from build123d import *

# Parameters (mm, degrees)
SKETCH1_W           = 50
SKETCH1_H           = 55
BOSS_EXTRUDE1_DEPTH = 5
SKETCH2_W           = 50
SKETCH2_H           = 70
BOSS_EXTRUDE2_DEPTH = 5
SKETCH3_W           = 50
SKETCH3_H           = 8
BOSS_EXTRUDE3_DEPTH = 50
FILLET1_R           = 2


with BuildPart() as part:
    # Sketch1 → Boss-Extrude1 (new body)
    with BuildSketch(Plane.XY):
        with Locations((-25, 27.5)):
            Rectangle(SKETCH1_W, SKETCH1_H)
    extrude(amount=BOSS_EXTRUDE1_DEPTH)

    # Sketch2 → Boss-Extrude2 (add)
    with BuildSketch(Plane(origin=(0, 0, 0), x_dir=(1, 0, 0), z_dir=(0, 1, 0))):
        with Locations((-25, -2.5)):
            Rectangle(SKETCH2_W, SKETCH2_H)
    extrude(amount=-BOSS_EXTRUDE2_DEPTH)

    # Sketch3 → Boss-Extrude3 (add)
    with BuildSketch(Plane(origin=(0, -5, 0), x_dir=(-1, 0, 0), z_dir=(0, -1, 0))):
        with Locations((25, -33.5)):
            Rectangle(SKETCH3_W, SKETCH3_H)
        with Locations((25, 28.5)):
            Rectangle(SKETCH3_W, SKETCH3_H)
    extrude(amount=BOSS_EXTRUDE3_DEPTH)

    # Fillet1
    fillet1_edges = [part.edges().sort_by_distance(p)[0] for p in [
        (-50, 0, 21.25),
        (-25, 0, 37.5),
        (0, 0, 21.25),
        (-50, -27.5, 37.5),
        (-50, -27.5, -32.5),
        (0, -27.5, -32.5),
        (0, -27.5, 37.5),
        (-50, 0, -16.25),
        (0, 0, -16.25),
        (-25, 0, -32.5),
        (0, -5, 2.5),
        (-50, -30, 29.5),
        (0, -55, 33.5),
        (0, -30, 29.5),
        (-25, -55, 37.5),
        (-25, -55, 29.5),
        (-50, -55, 33.5),
        (-50, -5, 2.5),
        (-25, -55, -24.5),
        (0, -30, -24.5),
        (-50, -55, -28.5),
        (-50, -30, -24.5),
        (-25, -55, -32.5),
        (0, -55, -28.5),
    ]]
    fillet(fillet1_edges, radius=FILLET1_R)


solid = part.part
Work out the finished part from the listing and answer in its coordinate system (mm). A direction names the side the tool comes from. Coordinates: 2 decimals unless noted, no trailing zeros. Write each loop counter-clockwise with the first axis right and the second up, starting at its lowest first coordinate (ties: lowest second). Pieces come first, ordered by that corner, then holes.
1. The part is cut by section A-A, the plane y = -20. Write down the section's boundary in (x, z), and give its area (3 significant figures).
Results list:
outline: (-50, -30.5) arc R2 ccw to (-48, -32.5) - (-2, -32.5) arc R2 ccw to (0, -30.5) - (0, -26.5) arc R2 ccw to (-2, -24.5) - (-48, -24.5) arc R2 ccw to (-50, -26.5) - close; (-50, 31.5) arc R2 ccw to (-48, 29.5) - (-2, 29.5) arc R2 ccw to (0, 31.5) - (0, 35.5) arc R2 ccw to (-2, 37.5) - (-48, 37.5) arc R2 ccw to (-50, 35.5) - close
area: 793 mm2
2. The part is cut by section D-D, the plane y = 45.5. Write down the section's boundary in (x, z).
Results list:
outline: (-50, 0) - (0, 0) - (0, 5) - (-50, 5) - close
3. Consider line 1 along Z through (x, y) = (-10, -29); line 2 along Z through (x, y) = (-21, 49.5); line 3 along Y through (x, z) = (-19, 2.5). Determine where each line is inside the solid, lowest interval first.
Results list:
line 1: z = -32.5 to -24.5, 29.5 to 37.5
line 2: z = 0 to 5
line 3: y = -5 to 55
4. The part is cut by section B-B, the plane x = -7.5. Write down the section's boundary in (y, z), and give its area (3 significant figures).
Results list:
outline: (-55, -30.5) arc R2 ccw to (-53, -32.5) - (-2, -32.5) arc R2 ccw to (0, -30.5) - (0, 0) - (55, 0) - (55, 5) - (0, 5) - (0, 35.5) arc R2 ccw to (-2, 37.5) - (-53, 37.5) arc R2 ccw to (-55, 35.5) - (-55, 31.5) arc R2 ccw to (-53, 29.5) - (-5, 29.5) - (-5, -24.5) - (-53, -24.5) arc R2 ccw to (-55, -26.5) - close
area: 1,420 mm2
5. For faces 1 (the flat face through (-25, -5, 2)), 2 (the flat face through (-25, 55, 2)), 3 (the flat face through (-25, 0, -15)), determine the directions among +Z, -Z, +X, -X, +Y, -Y from which every point of the face is accessible in a straight line to the end or side of a thin tool.
Results list:
face 1: +X, -X, -Y
face 2: +Z, -Z, +X, -X, +Y
face 3: -Z, +X, -X, +Y
6. The part is cut by section C-C, the plane z = -2. Write down the section's boundary in (x, y).
Results list:
outline: (-50, -3) arc R2 ccw to (-48, -5) - (-2, -5) arc R2 ccw to (0, -3) - (0, -2) arc R2 ccw to (-2, 0) - (-48, 0) arc R2 ccw to (-50, -2) - close
7. Flat-ended cylindrical pins translate along their axes: pin 1 (9 mm diameter, centred on x = -19.5, z = 14, fed in from +Y); pin 2 (2 mm diameter, centred on x = -43, y = 42.5, fed in from +Z); pin 3 (3 mm diameter, centred on y = -38, z = -24.5, fed in from -X). Find the tip coordinate at first contact, or state that the pin passes through.
Results list:
pin 1: stops at y = 0
pin 2: stops at z = 5
pin 3: stops at x = -49.94
8. For a pull along Z with two mould halves and no side action, classify faces 4 (the flat face through (-25, -29, -24.5)), 5 (the flat face through (-25, -27, -32.5)), 6 (the flat face through (-25, 0, 20)), 7 (the flat face through (-25, -27, 37.5)) as +Z half, -Z half, draft (parallel to the pull), parting line (faces both ways), or undercut.
Results list:
face 4: undercut
face 5: -Z half
face 6: draft
face 7: +Z half
